Autodesk Inventor part; units mm, degrees
ref_plane "YZ Plane" through (0, 0, 0) normal (1, 0, 0) x (0, 1, 0)
ref_plane "XZ Plane" through (0, 0, 0) normal (0, 1, 0) x (-1, 0, 0)
ref_plane "XY Plane" through (0, 0, 0) normal (0, 0, 1) x (1, 0, 0)
sketch "Sketch1" plane through (0, 0, 0) normal (0, 1, 0) x (-1, 0, 0)
  line L0 (0, -55.88) -> (-12.7, -55.88)
  line L1 (-12.7, 0) -> (0, 0)
  line L2 (0, 0) -> (0, -20.94)
  line L3 (0, -34.94) -> (0, -55.88)
  line L4 (-12.7, -55.88) -> (-12.7, -34.94)
  line L5 (-12.7, -20.94) -> (-12.7, 0)
  line L6 (0, -20.94) -> (0, -34.94)
  line L7 (-12.7, -20.94) -> (-12.7, -34.94)
  dimension "d1" = 55.88
  dimension "d2" = 12.7
extrude "Extrusion1" add sketch "Sketch1" along normal blind 1.5
sketch "Sketch2" plane through (0, 1.5, 0) normal (0, 1, 0) x (1, 0, 0)
  line L0 (12.7, 0) -> (12.7, 55.88)
  line L1 (12.7, 0) -> (10.16, 0)
  line L2 (12.7, 2.54) -> (12.7, 0)
  circle A0 centre (10.16, 2.54) radius 1.092
  circle A1 centre (10.16, 53.34) radius 1.092
  point P0 (0, 0)
  dimension "d8" = 2.184
  dimension "d10" = 2.184
extrude "Extrusion2" cut sketch "Sketch2" against normal blind 1.5
sketch "Sketch5" plane through (0, 0, 0) normal (0, 0, 1) x (1, 0, 0)
  line L0 (12.7, 0) -> (0, 0)
  line L1 (6.35, 0) -> (6.35, 1.5)
  line L2 (12.7, 1.5) -> (0, 1.5)
  line L3 (0, 0) -> (0, 1.5)
  line L4 (0, 0.75) -> (12.7, 0.75)
  line L5 (12.7, 0) -> (12.7, 1.5)
  circle A0 centre (6.35, 0.75) radius 5.175
  dimension "d30" = 10.35
extrude "Extrusion5" add sketch "Sketch5" along normal blind 2 contours A0 L0 | L0 L1 L4 A0 | L0 A0 L4 L1 | L4 L1 L2 A0 | L4 A0 L2 L1 | L2 A0
sketch "Sketch6" plane through (6.35, 0.75, 2) normal (0, 0, 1) x (1, 0, 0)
  circle A0 centre (0, 0) radius 5.175
  circle A1 centre (0, 0) radius 3.175
  point P0 (-6.35, -0.75)
  dimension "d35" = 6.35
extrude "Extrusion6" add sketch "Sketch6" along normal blind 9
sketch "Sketch7" plane through (12.7, 0, -55.88) normal (0, 0, -1) x (-1, 0, 0)
  line L0 (0, 0) -> (0, 1.5)
  line L1 (0, 0.75) -> (12.7, 0.75)
  line L2 (12.7, 0) -> (12.7, 1.5)
  line L3 (11.4704, 1.5) -> (1.2296, 1.5)
  line L4 (6.35, 1.5) -> (6.35, 0)
  circle A0 centre (6.35, 0.75) radius 5.175
extrude "Extrusion7" add sketch "Sketch7" along normal blind 2
sketch "Sketch8" plane through (6.35, 0.75, -57.88) normal (0, 0, -1) x (-1, 0, 0)
  circle A0 centre (0, 0) radius 5.175
  circle A1 centre (0, 0) radius 3.175
  point P0 (6.35, -0.75)
  dimension "d40" = 6.35
extrude "Extrusion8" add sketch "Sketch8" along normal blind 9
thread "Thread1"
thread "Thread2"
sketch "Sketch9" plane through (0, 0, 0) normal (0, 0, -1) x (-1, 0, 0)
  arc A0 (-11.4704, 0) -> (-1.2296, 0) centre (-6.35, 0.75) ccw
  line L0 (0, 0) -> (-1.2296, 0)
  line L1 (-11.4704, 0) -> (-1.2296, 0)
  circle A1 centre (-6.35, 0.75) radius 5.175
extrude "Extrusion9" add sketch "Sketch9" along normal up to next contours L1 A0
sketch "Sketch10" plane through (10.16, 0, -2.54) normal (0, 1, 0) x (1, 0, 0)
  circle A0 centre (0, 0) radius 1.092
  circle A1 centre (0, 50.8) radius 1.092
  circle A2 centre (0, 50.8) radius 1.092
  point P0 (-10.16, -2.54)
  dimension "d60" = 2.184
extrude "Extrusion10" cut sketch "Sketch10" against normal up to next
sketch "Sketch12" plane through (0, 1.5, 0) normal (0, 1, 0) x (1, 0, 0)
  circle A0 centre (10.16, 2.54) radius 1.092
  circle A1 centre (10.16, 2.54) radius 1.092
  circle A2 centre (10.16, 2.54) radius 2.2225
  circle A3 centre (10.16, 53.34) radius 1.092
  circle A4 centre (10.16, 53.34) radius 1.092
  circle A5 centre (10.16, 53.34) radius 2.2225
  point P0 (0, 0)
  dimension "d54" = 4.445
  dimension "d55" = 4.445
extrude "Extrusion11" cut sketch "Sketch12" against normal blind 5.925
sketch "Sketch13" plane through (0, 1.5, 0) normal (0, 1, 0) x (1, 0, 0)
  line L0 (12.7, 0) -> (12.7, 55.88)
  line L1 (12.7, 55.88) -> (0, 55.88)
  line L2 (0, 55.88) -> (0, 0)
  line L3 (0, 0) -> (12.7, 0)
  line L4 (12.7, 0) -> (12.7, 55.88)
  circle A0 centre (10.16, 53.34) radius 1.092
  circle A1 centre (10.16, 53.34) radius 1.092
  circle A2 centre (10.16, 2.54) radius 1.092
  circle A3 centre (10.16, 2.54) radius 1.092
extrude "Extrusion12" add sketch "Sketch13" along normal blind 10.4775
thread "Thread5"
thread "Thread6"
sketch "Sketch14" plane through (10.16, 1.5, -53.34) normal (0, -1, 0) x (1, 0, 0)
  circle A0 centre (0, 0) radius 1.092
  circle A1 centre (0, 0) radius 2.2225
  circle A2 centre (0, 50.8) radius 2.2225
  circle A3 centre (0, 50.8) radius 2.2225
  circle A4 centre (0, 0) radius 1.092
  circle A5 centre (0, 50.8) radius 1.092
  point P0 (-10.16, 53.34)
extrude "Extrusion13" cut sketch "Sketch14" against normal blind 1
sketch "Sketch15" plane through (0, 11.9775, 0) normal (0, 1, 0) x (1, 0, 0)
  line L0 (12.7, 0) -> (12.7, 6.985)
  line L1 (12.7, 0) -> (12.7, 55.88)
  line L2 (12.7, 0) -> (19.685, 0) construction
  line L3 (11.525, -11) -> (11.525, 66.88)
  line L4 (11.43, 6.985) -> (13.97, 6.985) construction
  line L5 (11.43, 6.985) -> (12.43, 6.985) construction
  line L6 (11.43, 9.525) -> (12.43, 9.525) construction
  line L7 (12.7, 5.985) -> (12.7, 10.525)
  line L8 (12.7, 5.985) -> (12.7, 5.485)
  line L9 (12.7, 5.485) -> (9.93, 5.485)
  line L10 (9.93, 5.485) -> (9.93, 11.025)
  line L11 (9.93, 11.025) -> (12.7, 11.025)
  line L12 (12.7, 11.025) -> (12.7, 10.525)
  point P0 (0, 0)
  dimension "d72" = 90
  dimension "d130" = 0.5
  dimension "d131" = 2.77
  dimension "d132" = 5.54
extrude "Extrusion14" cut sketch "Sketch15" against normal blind 8
sketch "Sketch16" plane through (0, 11.9775, 0) normal (0, 1, 0) x (1, 0, 0)
  line L0 (12.7, 0) -> (12.7, 55.88)
  line L1 (12.7, 40.234) -> (13.97, 40.234) construction
  line L2 (0, 0) -> (12.7, 0)
  line L3 (11.43, 0) -> (40.005, 0) construction
  line L4 (11.525, -11) -> (11.525, 66.88)
  line L5 (11.43, 28.575) -> (13.97, 28.575) construction
  line L6 (11.43, 46.355) -> (12.43, 46.355) construction
  line L7 (11.43, 28.575) -> (13.97, 28.575) construction
  line L8 (11.43, 20.955) -> (12.43, 20.955) construction
  line L9 (6.89, 19.955) -> (6.89, 47.355)
  line L10 (12.7, 47.355) -> (12.7, 19.955)
  line L11 (6.89, 47.355) -> (6.89, 47.855)
  line L12 (6.89, 47.855) -> (12.7, 47.855)
  line L13 (12.7, 47.855) -> (12.7, 47.355)
  line L14 (12.7, 19.955) -> (12.7, 19.455)
  line L15 (12.7, 0) -> (12.7, 55.88)
  line L16 (12.7, 19.455) -> (6.89, 19.455)
  line L17 (6.89, 19.455) -> (6.89, 19.955)
  point P0 (12.7, 10.525)
  dimension "d123" = 5.81
  dimension "d129" = 28.4
extrude "Extrusion15" cut sketch "Sketch16" against normal blind 8 contours L16 L4 L12 L0 | L16 L17 L9 L11 L12 L4
properties part number "Line Sensor 6 Bracket"
Verification items for the finished model (mm, model axes). A direction names the side the tool comes from. Give positions to 0.01 mm unless a question says otherwise; leave off trailing zeros. Order: outer loops, then holes, each group sorted by start corner. A loop starts at its lowest first (then second) coordinate and runs counter-clockwise, first axis right, second up. Notation, with made-up numbers: M 6,26.5 L 58,26.5 A22 ccw 58,56.5 Z; hole C -3.75,69 d3. An arc over 180 degrees is marked long. Answer as a JSON object with one key per item and string values. Group by question number.
1) Cross-section at D-D (x = 4.25). Enter the section's corners in (y, z).
2) Depth check by flat-ended pin: pin 1 Ø4 at (x, y) = (6.35, 0.75) entering from +Z; pin 2 Ø2 at (x, z) = (11, -54) entering from -Y; pin 3 Ø2 at (x, y) = (11.5, 7) entering from -Z. Enter the tip coordinate at first touch or a pass-through.
3) Cross-section at A-A (z = -2.54). Enter the section's corners in (x, y), then the cut area to 3 significant figures.
4) Access from +Z, -Z, +X, -X, +Y, -Y to the whole of each face (thin tool, end or side, straight path). Record for faces 1 (the face through (6, 7, 0)), 2 (the face through (6, 1, 2)), 3 (the face through (9.93, 8, -8)).
5) Mould release check, pull along Y, two halves, no side actions. Record for faces 4 (the face through (11.286, -0.804, 5.423)), 5 (the face through (7.94, -0.05, -53.44)), 6 (the face through (3.18, 0.61, 6.44)): released by +Y, released by -Y, zero draft, split by the parting line, or undercut.
6) Scan lines: line 1 along Z through (x, y) = (11.5, 7.25) (3 decimals); line 2 along Z through (x, y) = (10.16, 7.75) (3 decimals); line 3 along Z through (x, y) = (10.25, 5) (3 decimals). Record each from-to range of solid material in increasing order. Write a range as [from, to].
7) Cross-section at C-C (z = -27.5). Enter the section's corners in (x, y), then the cut area to 3 significant figures.
8) Cross-section at B-B (y = 0.75). Enter the section's corners in (x, z) (1 decimal), then the cut area to 3 significant figures.
Result sheet:
{
 "1": {"outline": "M -3.98,-66.88 L -1.63,-66.88 L -1.63,-57.88 L 3.13,-57.88 L 3.13,-66.88 L 5.48,-66.88 L 5.48,-55.88 L 11.98,-55.88 L 11.98,0 L 5.48,0 L 5.48,11 L 3.13,11 L 3.13,2 L -1.63,2 L -1.63,11 L -3.98,11 L -3.98,-55.88 Z"},
 "2": {"pin 1": "stops at z = 2", "pin 2": "stops at y = 2.5", "pin 3": "stops at z = -55.88"},
 "3": {"outline": "M 0,0 L 1.23,0 A5.18 ccw 7.94,-4.18 L 7.94,2.5 L 9.07,2.5 L 9.07,11.98 L 0,11.98 Z; M 11.25,2.5 L 12.38,2.5 L 12.38,0 L 12.7,0 L 12.7,11.98 L 11.25,11.98 Z", "area": "144 mm2"},
 "4": {"face 1": "+Z, +Y", "face 2": "+Z", "face 3": "+X, +Y"},
 "5": {"face 4": "split by the parting line", "face 5": "zero draft", "face 6": "undercut"},
 "6": {"line 1": "z = [-55.88, -47.855], [-19.455, -11.025], [-5.485, 0]", "line 2": "z = [-55.88, -54.432], [-52.248, -47.855], [-19.455, -11.025], [-5.485, -3.632], [-1.448, 0]", "line 3": "z = [-55.88, -54.428], [-52.252, -47.855], [-19.455, -11.025], [-5.485, -3.628], [-1.452, 0]"},
 "7": {"outline": "M 0,0 L 1.23,0 A5.18 ccw 11.47,0 L 12.7,0 L 12.7,3.98 L 6.89,3.98 L 6.89,11.98 L 0,11.98 Z", "area": "140 mm2"},
 "8": {"outline": "M 0,-55.9 L 1.2,-55.9 L 1.2,-66.9 L 3.2,-66.9 L 3.2,-57.9 L 9.5,-57.9 L 9.5,-66.9 L 11.5,-66.9 L 11.5,-55.9 L 12.7,-55.9 L 12.7,0 L 11.5,0 L 11.5,11 L 9.5,11 L 9.5,2 L 3.2,2 L 3.2,11 L 1.2,11 L 1.2,0 L 0,0 Z; hole C 10.2,-53.3 d4.4; hole C 10.2,-2.5 d4.4", "area": "792 mm2"}
}
